Can you work these out from the drawing? Everything is in mm from the part's minimum corner. A direction names the side the tool comes from. Round coordinates to 2 decimals unless told otherwise and drop trailing zeros. Loops run counter-clockwise (first coordinate to the right, second up) from the corner with the lowest first, then second, coordinate; pieces in that order, holes last. Notation, with made-up numbers: (-13, -20.5) -> (-3, -20.5) arc R4 ccw to (-3, -13.5) -> close; hole circle Ø5 at (55, 5). An arc over 180 degrees is marked (long way). One line per item, written item: value.
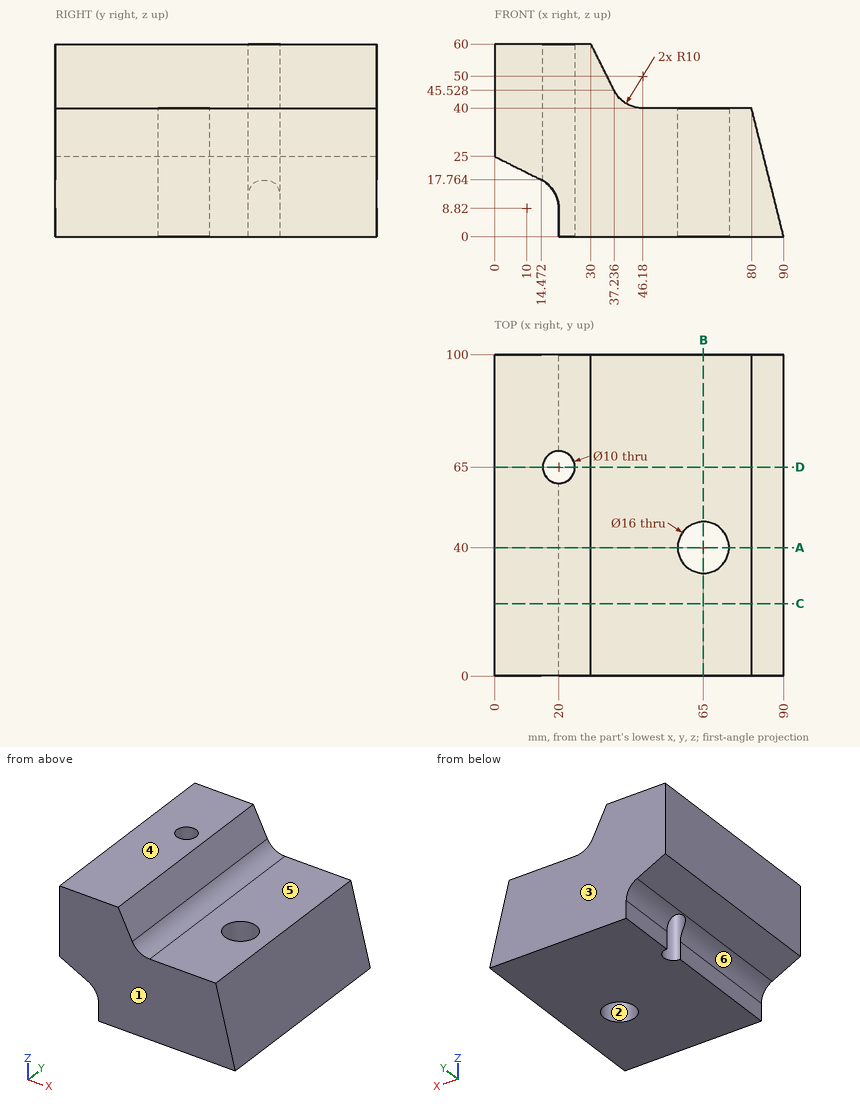
Item 1: If we section it at C-C on y = 22.5: List the corners of the cut face in (x, z) for me, plus the area to 3 significant figures.
Output:
outline: (0, 25) -> (14.47, 17.76) arc R10 cw to (20, 8.82) -> (20, 0) -> (90, 0) -> (80, 40) -> (46.18, 40) arc R10 cw to (37.24, 45.53) -> (30, 60) -> (0, 60) -> close
area: 3,710 mm²
Item 2: Will these pins go through, and if not, where does the flat tip stop? pin 1 Ø2 at (y, z) = (43, 34) entering from +X; pin 2 Ø7 at (y, z) = (85, 4) entering from -X; pin 3 Ø5 at (y, z) = (61.5, 23) entering from +X (1 decimal); pin 4 Ø13 at (x, y) = (65, 40) entering from -Z.
Output:
pin 1: stops at x = 81.75
pin 2: stops at x = 20
pin 3: stops at x = 84.9
pin 4: passes through
Item 3: If we section it at D-D on y = 65: List the corners of the cut face in (x, z) for me, plus the area to 3 significant figures.
Output:
outline: (0, 25) -> (14.47, 17.76) arc R10 cw to (15, 17.48) -> (15, 60) -> (0, 60) -> close; (25, 0) -> (90, 0) -> (80, 40) -> (46.18, 40) arc R10 cw to (37.24, 45.53) -> (30, 60) -> (25, 60) -> close
area: 3,190 mm²
Item 4: For the marked faces 5 and 6, which set-ups out of +Z, -Z, +X, -X, +Y, -Y let a thin tool reach every point of the face, with its end or its side?
Output:
face 5: +Z, +X, +Y, -Y
face 6: -Z, -X, +Y, -Y
Item 5: If we section it at A-A on y = 40: List the corners of the cut face in (x, z) for me.
Output:
outline: (0, 25) -> (14.47, 17.76) arc R10 cw to (20, 8.82) -> (20, 0) -> (57, 0) -> (57, 40) -> (46.18, 40) arc R10 cw to (37.24, 45.53) -> (30, 60) -> (0, 60) -> close; (73, 0) -> (90, 0) -> (80, 40) -> (73, 40) -> close
Item 6: If we mould it in two halves opening along Y, with no side actions, what happens to the marked faces 1, 2, 3 and 4? For each: released by +Y, released by -Y, zero draft, split by the parting line, or undercut.
Output:
face 1: released by -Y
face 2: undercut
face 3: released by +Y
face 4: zero draft
Item 7: I need wall thicknesses on line 1 (Y direction, x = 20, z = 24); line 2 (Y direction, x = 65, z = 31); line 3 (Z direction, x = 78, y = 8.5). Which ranges of each line are inside material? Lowest first, please. Write a range as from..to.
Output:
line 1: y = 0..60, 70..100
line 2: y = 0..32, 48..100
line 3: z = 0..40
Item 8: If we section it at B-B on x = 65: List the corners of the cut face in (y, z) for me.
Output:
outline: (0, 0) -> (32, 0) -> (32, 40) -> (0, 40) -> close; (48, 0) -> (100, 0) -> (100, 40) -> (48, 40) -> close
